Could you check a few things on this model? Use its own coordinates, in mm. Face numbers are marked on the shaded views. Give positions to 0.01 mm unless a question says otherwise; leave off trailing zeros. Order: outer loops, then holes, each group sorted by start corner. A loop starts at its lowest first (then second) coordinate and runs counter-clockwise, first axis right, second up.
(1) If we mould it in two halves opening along Y, with no side actions, what happens to the marked faces 1, 2 and 3? For each: released by +Y, released by -Y, zero draft, split by the parting line, or undercut.
(2) Imagine slicing it at B-B, the plane x = -114.3. Write out the boundary of the cut face in (y, z) (3 decimals).
(3) If I drill on probe 1 along Y at (x, z) = (114.3, -11); probe 2 along Y at (x, z) = (-114.3, -52.9), over which ranges is the centre line in solid material (lowest first)?
(4) Will these pins go through, and if not, where does the flat tip stop? pin 1 (7.5 mm diameter, centred on x = -114.3, y = -114.3, fed in from -Z); pin 2 (1 mm diameter, centred on x = -64.5, y = -51, fed in from +Z); pin 3 (4 mm diameter, centred on x = -114.3, y = 114.3, fed in from -Z); pin 4 (9 mm diameter, centred on x = -113.5, y = 115.5, fed in from +Z).
(5) Imagine slicing it at A-A, the plane y = 0. Write out the boundary of the cut face in (x, z), then the cut area to 3 significant figures.
(6) Imagine slicing it at C-C, the plane z = -45. Write out the boundary of the cut face in (x, y).
from build123d import *

# Parameters (mm, degrees)
SKETCH1_W                                     = 254
SKETCH1_H                                     = 254
SKETCH1_R                                     = 25.4
BOSS_EXTRUDE1_DEPTH                           = 57.15
CBORE_FOR_1_4_SOCKET_HEAD_CAP_SCREW2_AT_COUNT = 2
CBORE_FOR_1_4_SOCKET_HEAD_CAP_SCREW2_AT_PITCH = 228.6
CBORE_FOR_1_4_SOCKET_HEAD_CAP_SCREW2_2_COUNT  = 2
CBORE_FOR_1_4_SOCKET_HEAD_CAP_SCREW2_2_PITCH  = 323.289220358
CBORE_FOR_1_4_SOCKET_HEAD_CAP_SCREW2_3_COUNT  = 2
CBORE_FOR_1_4_SOCKET_HEAD_CAP_SCREW2_3_PITCH  = 228.6
F_10_32_TAPPED_HOLE1_D                        = 4.0386
F_10_32_TAPPED_HOLE1_DEPTH                    = 19.05
F_10_32_TAPPED_HOLE1_TIP                      = 1.213317848


with BuildPart() as part:
    # Sketch1 → Boss-Extrude1 (new body)
    with BuildSketch(Plane.XY):
        Rectangle(SKETCH1_W, SKETCH1_H)
        Circle(SKETCH1_R, mode=Mode.SUBTRACT)
    extrude(amount=-BOSS_EXTRUDE1_DEPTH)

    # Sketch3 → CBORE for 1/4 Socket Head Cap Screw2 (revolve, cut)
    with BuildSketch(Plane(origin=(-114.3, 114.3, 0), x_dir=(0, -1, 0), z_dir=(1, 0, 0))):
        Polygon((0, 0), (0, 57.15), (3.8989, 57.15), (3.2639, 56.515), (3.2639, 50.8), (5.55625, 50.8), (5.55625, 0.635), (6.19125, 0), align=None)
    cbore_for_1_4_socket_head_cap_screw2 = revolve(axis=Axis((-114.3, 114.3, 6.35), (0, 0, -1)), mode=Mode.SUBTRACT)

    # CBORE for 1/4 Socket Head Cap Screw2 at: CBORE for 1/4 Socket Head Cap Screw2 ×2
    with Locations(*[(i * CBORE_FOR_1_4_SOCKET_HEAD_CAP_SCREW2_AT_PITCH, 0, 0) for i in range(1, CBORE_FOR_1_4_SOCKET_HEAD_CAP_SCREW2_AT_COUNT)]):
        add(cbore_for_1_4_socket_head_cap_screw2, mode=Mode.SUBTRACT)

    # CBORE for 1_4 Socket Head Cap Screw2 2: CBORE for 1/4 Socket Head Cap Screw2 ×2
    with Locations(*[Vector(0.707106781, -0.707106781, 0) * (i * CBORE_FOR_1_4_SOCKET_HEAD_CAP_SCREW2_2_PITCH) for i in range(1, CBORE_FOR_1_4_SOCKET_HEAD_CAP_SCREW2_2_COUNT)]):
        add(cbore_for_1_4_socket_head_cap_screw2, mode=Mode.SUBTRACT)

    # CBORE for 1_4 Socket Head Cap Screw2 3: CBORE for 1/4 Socket Head Cap Screw2 ×2
    with Locations(*[(0, -i * CBORE_FOR_1_4_SOCKET_HEAD_CAP_SCREW2_3_PITCH, 0) for i in range(1, CBORE_FOR_1_4_SOCKET_HEAD_CAP_SCREW2_3_COUNT)]):
        add(cbore_for_1_4_socket_head_cap_screw2, mode=Mode.SUBTRACT)

    # #10-32 Tapped Hole1
    with Locations(Plane(origin=(0, -127, 0), x_dir=(-1, 0, 0), z_dir=(0, -1, 0))):
        with Locations((3.175, 25.4), (-9.525, 25.4), (37, 14.2875), (37, 36.5125)):
            Hole(F_10_32_TAPPED_HOLE1_D / 2, depth=F_10_32_TAPPED_HOLE1_DEPTH)
            with Locations((0, 0, -(F_10_32_TAPPED_HOLE1_DEPTH + F_10_32_TAPPED_HOLE1_TIP / 2))):  # 118° drill point
                Cone(0, F_10_32_TAPPED_HOLE1_D / 2, F_10_32_TAPPED_HOLE1_TIP, mode=Mode.SUBTRACT)


solid = part.part
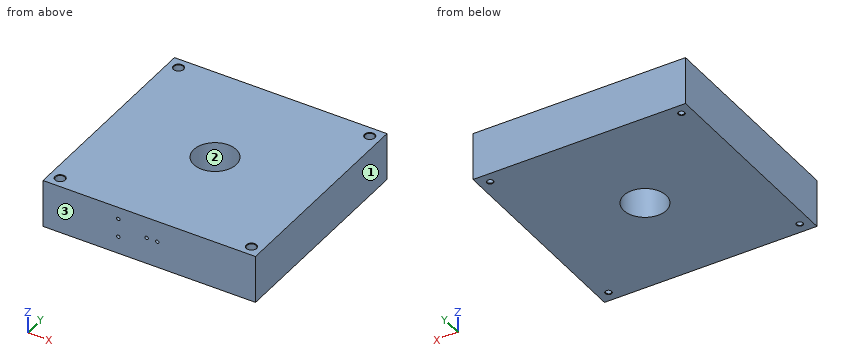
Answer block:
1. face 1: zero draft
1. face 2: undercut
1. face 3: released by -Y
2. outline: (-127, -57.15) - (-118.199, -57.15) - (-117.564, -56.515) - (-117.564, -50.8) - (-119.856, -50.8) - (-119.856, -0.635) - (-120.491, 0) - (-127, 0) - close; (-111.036, -56.515) - (-110.401, -57.15) - (110.401, -57.15) - (111.036, -56.515) - (111.036, -50.8) - (108.744, -50.8) - (108.744, -0.635) - (108.109, 0) - (-108.109, 0) - (-108.744, -0.635) - (-108.744, -50.8) - (-111.036, -50.8) - close; (117.564, -56.515) - (118.199, -57.15) - (127, -57.15) - (127, 0) - (120.491, 0) - (119.856, -0.635) - (119.856, -50.8) - (117.564, -50.8) - close
3. probe 1: y = -127 to -119.86, -108.74 to 108.74, 119.86 to 127
3. probe 2: y = -127 to -117.56, -111.04 to 111.04, 117.56 to 127
4. pin 1: stops at z = -57
4. pin 2: stops at z = 0
4. pin 3: passes through
4. pin 4: stops at z = -0.25
5. outline: (-127, -57.15) - (-25.4, -57.15) - (-25.4, 0) - (-127, 0) - close; (25.4, -57.15) - (127, -57.15) - (127, 0) - (25.4, 0) - close
5. area: 11,600 mm2
6. outline: (-127, -127) - (127, -127) - (127, 127) - (-127, 127) - close; hole circle Ø11.11 at (-114.3, -114.3); hole circle Ø11.11 at (-114.3, 114.3); hole circle Ø50.8 at (0, 0); hole circle Ø11.11 at (114.3, -114.3); hole circle Ø11.11 at (114.3, 114.3)
